Here's how the part is built. I have some questions about the finished solid (model axes, mm). Face numbers are marked on the shaded views. A direction names the side the tool comes from. Coordinates: 2 decimals unless noted, no trailing zeros. Loops run counter-clockwise (first coordinate to the right, second up) from the corner with the lowest first, then second, coordinate; pieces in that order, holes last.
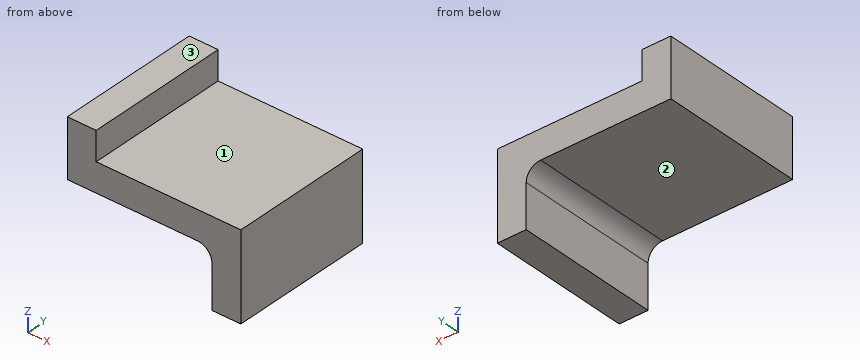
from build123d import *

# Parameters (mm, degrees)
F1_DEPTH = 25


with BuildPart() as f1:
    # F0 (on Front) → F1 (new body)
    with BuildSketch(Plane.XZ):
        with BuildLine():
            Line((-2.626851, 0), (-2.5, 0))
            ThreePointArc((-2.5, 0), (-0.732233, -0.732233), (0, -2.5))
            Line((0, -2.5), (0, -10))
            Line((0, -10), (5, -10))
            Line((5, -10), (5, 5))
            Line((5, 5), (-20, 5))
            Line((-20, 5), (-20, 10))
            Line((-20, 10), (-25, 10))
            Line((-25, 10), (-25, 0))
            Line((-25, 0), (-2.626851, 0))
        make_face()
    extrude(amount=F1_DEPTH)


solid = f1.part
Q1. Suppose I cut it at A-A on y = -14.75. Write out the boundary of the cut face in (x, z).
Q2. Please list where these lines run through material, in increasing order: probe 1 along Z at (x, y) = (-20.75, -15.25); probe 2 along X at (y, z) = (-15.25, 9); probe 3 along X at (y, z) = (-15.5, -5.5).
Q3. For the marked faces 1, 2 and 3, which set-ups out of +Z, -Z, +X, -X, +Y, -Y let a thin tool reach every point of the face, with its end or its side?
Q4. Suppose I cut it at B-B on x = 1. Write out the boundary of the cut face in (y, z), and give its area (3 significant figures).
Q5. Will these pins go through, and if not, where does the flat tip stop? P1, Ø4, axis at y = -16, z = 8.5, coming from the +X side; P2, Ø6, axis at x = -2.5, y = -20, coming from the +Z side; P3, Ø8, axis at y = -8, z = -5.5, coming from the -X side.
Q6. Suppose I cut it at C-C on z = -5.5. Write out the boundary of the cut face in (x, y), and give its area (3 significant figures).
Check values:
1. outline: (-25, 0) - (-2.5, 0) arc R2.5 cw to (0, -2.5) - (0, -10) - (5, -10) - (5, 5) - (-20, 5) - (-20, 10) - (-25, 10) - close
2. probe 1: z = 0 to 10
2. probe 2: x = -25 to -20
2. probe 3: x = 0 to 5
3. face 1: +Z, +X, +Y, -Y
3. face 2: -Z, -X, +Y, -Y
3. face 3: +Z, +X, -X, +Y, -Y
4. outline: (-25, -10) - (0, -10) - (0, 5) - (-25, 5) - close
4. area: 375 mm2
5. P1: stops at x = -20
5. P2: stops at z = 5
5. P3: stops at x = -0.21
6. outline: (0, -25) - (5, -25) - (5, 0) - (0, 0) - close
6. area: 125 mm2
